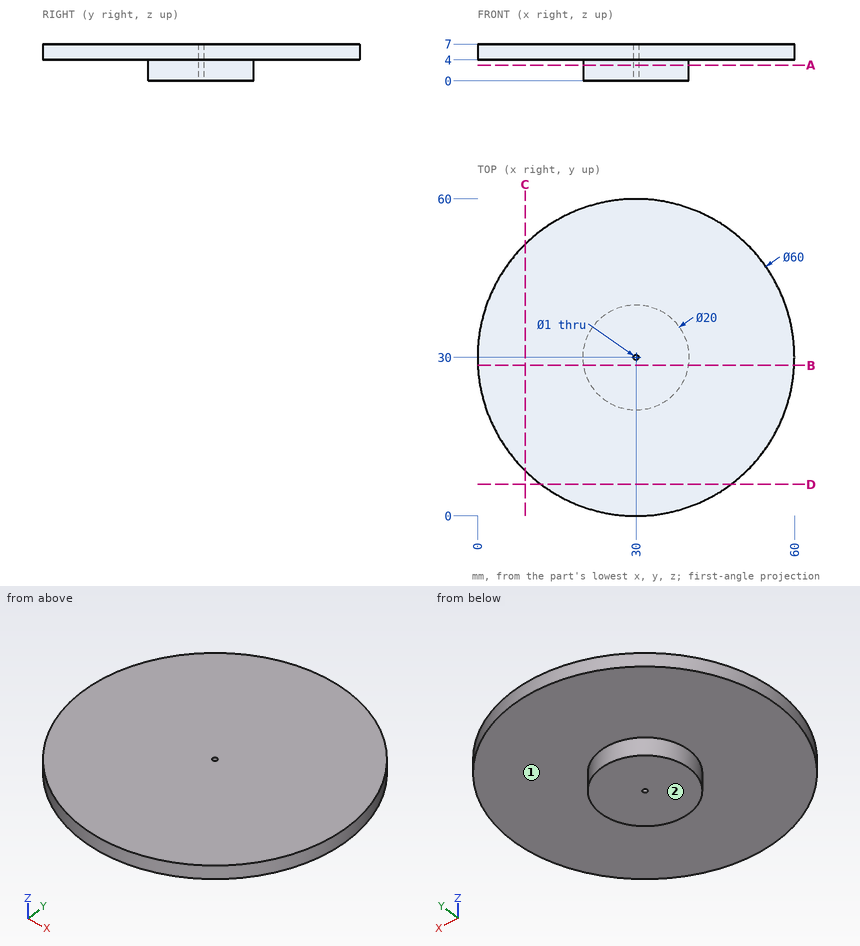
The figure shows three views and two pictorial views of one solid part (mm, origin at its lowest corner). Answer the questions. A direction names the side the tool comes from. Round coordinates to 2 decimals unless told otherwise and drop trailing zeros. Loops run counter-clockwise (first coordinate to the right, second up) from the corner with the lowest first, then second, coordinate; pieces in that order, holes last. Notation, with made-up numbers: M 28.25,2 L 66.25,2 A31 ccw 66.25,34 Z; hole C 12.5,29.25 d6. An arc over 180 degrees is marked long. Write each question's results on one line, items separated by ' | '. Start each with the question number.
1) Which of the six approach directions +Z, -Z, +X, -X, +Y, -Y give full straight-line access (tool end or side, diameter ignored) to the marked faces 1 and 2?
2) Find section D-D on y = 6. Write down the section's boundary in (x, z).
3) Find section C-C on x = 9. Write down the section's boundary in (y, z), plus the area to 3 significant figures.
4) Find section B-B on y = 28.5. Write down the section's boundary in (x, z).
5) Straight lines are drawn through the part: probe 1 along Z at (x, y) = (17, 12); probe 2 along Y at (x, z) = (30, 3); probe 3 along Y at (x, z) = (25, 1). For each, find the intervals that lie inside material, in ascending order.
6) Find section A-A on z = 3. Write down the section's boundary in (x, y).
7) This flat-tipped pin is pushed along its axis until it touches: pin 1 (2 mm diameter, centred on x = 34.5, y = 18, fed in from -Z). Where does it stop, or does it pass through?
Final values:
1) face 1: -Z | face 2: -Z, +X, -X, +Y, -Y
2) outline: M 12,4 L 48,4 L 48,7 L 12,7 Z
3) outline: M 8.58,4 L 51.42,4 L 51.42,7 L 8.58,7 Z | area: 129 mm²
4) outline: M 0.04,4 L 20.11,4 L 20.11,0 L 39.89,0 L 39.89,4 L 59.96,4 L 59.96,7 L 0.04,7 Z
5) probe 1: 4 to 7 | probe 2: 20 to 29.5, 30.5 to 40 | probe 3: 21.34 to 38.66
6) outline: C 30,30 d20; hole C 30,30 d1
7) pin 1: z = 4
